Geometry: see drawing. Coordinates: mm, zero at the bounding-box minimum. A direction names the side the tool comes from. Coordinates: 2 decimals unless noted, no trailing zeros. Order: outer loops, then holes, each group sorted by start corner. A loop starts at its lowest first (then second) coordinate and runs counter-clockwise, first axis right, second up.
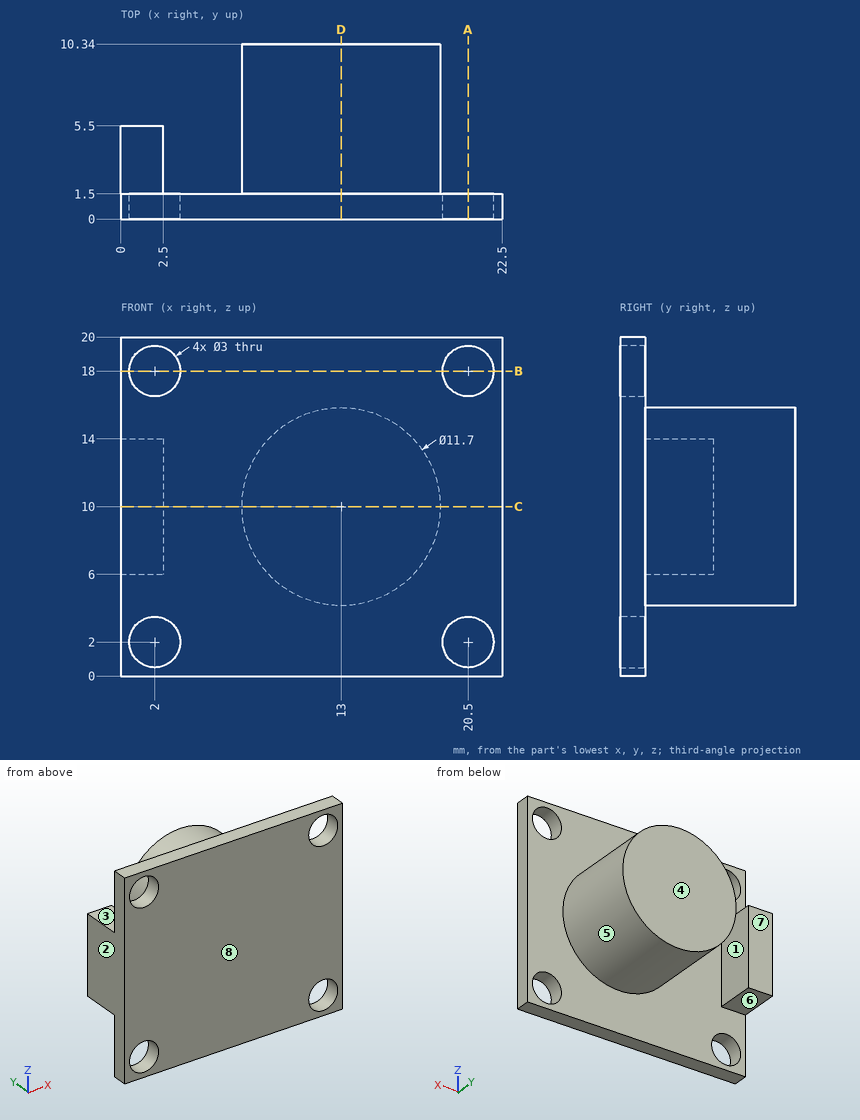
Q1. Material intervals for line 1 along X through (y, z) = (0.9, 18); line 2 along Y through (x, z) = (5, 1.5); line 3 along Z through (x, y) = (12.75, 3), sorted ascending.
Solutions:
line 1: x = 0 to 0.5, 3.5 to 19, 22 to 22.5
line 2: y = 0 to 1.5
line 3: z = 4.16 to 15.84
Q2. Section query D-D on x = 13. Output: boundary loops of the cut face in (y, z).
Solutions:
outline: (0, 0) - (1.5, 0) - (1.5, 4.15) - (10.34, 4.15) - (10.34, 15.85) - (1.5, 15.85) - (1.5, 20) - (0, 20) - close
Q3. Section query B-B on z = 18. Output: boundary loops of the cut face in (x, y).
Solutions:
outline: (0, 0) - (0.5, 0) - (0.5, 1.5) - (0, 1.5) - close; (3.5, 0) - (19, 0) - (19, 1.5) - (3.5, 1.5) - close; (22, 0) - (22.5, 0) - (22.5, 1.5) - (22, 1.5) - close
Q4. Pull-direction query (X, two-part tool) for the marked faces 1, 2 and 3; classes: pulls with the +X half, pulls with the -X half, needs draft (parallel to the pull), parting line crosses it, or undercut.
Solutions:
face 1: undercut
face 2: pulls with the -X half
face 3: needs draft
Q5. Set-up query: the marked faces 4, 5, 6, 7 and 8. Return all of +Z, -Z, +X, -X, +Y, -Y with unobstructed straight access to the full face (end or side cutting, diameter ignored); none if empty.
Solutions:
face 4: +Z, -Z, +X, -X, +Y
face 5: +Y
face 6: -Z, -X, +Y
face 7: +Z, -Z, -X, +Y
face 8: +Z, -Z, +X, -X, -Y
Q6. Section query A-A on x = 20.5. Output: boundary loops of the cut face in (y, z), plus the area to 3 significant figures.
Solutions:
outline: (0, 0) - (1.5, 0) - (1.5, 0.5) - (0, 0.5) - close; (0, 3.5) - (1.5, 3.5) - (1.5, 16.5) - (0, 16.5) - close; (0, 19.5) - (1.5, 19.5) - (1.5, 20) - (0, 20) - close
area: 21.0 mm2
Q7. Section query C-C on z = 10. Output: boundary loops of the cut face in (x, y), plus the area to 3 significant figures.
Solutions:
outline: (0, 0) - (22.5, 0) - (22.5, 1.5) - (18.85, 1.5) - (18.85, 10.34) - (7.15, 10.34) - (7.15, 1.5) - (2.5, 1.5) - (2.5, 5.5) - (0, 5.5) - close
area: 147 mm2
Q8. Pin query (flat end, axial travel): P1, Ø1.2, axis at x = 1, y = 2.5, coming from the +Z side; P2, Ø3, axis at y = 3.5, z = 9.5, coming from the +X side; P3, Ø0.8, axis at x = 1.5, z = 8.5, coming from the +Y side. Return the tip coordinate at first contact, or that it passes through.
Solutions:
P1: stops at z = 14
P2: stops at x = 18.85
P3: stops at y = 5.5
